The figure shows three views and two pictorial views of one solid part (mm, origin at its lowest corner). Answer the questions. A direction names the side the tool comes from. Round coordinates to 2 decimals unless told otherwise and drop trailing zeros. Write each loop counter-clockwise with the first axis right and the second up, starting at its lowest first coordinate (ties: lowest second). Pieces come first, ordered by that corner, then holes. Notation, with made-up numbers: (56, 46) - (72, 46) arc R16 ccw to (72, 50) - close; hole circle Ø2 at (73, -23). An arc over 180 degrees is marked (long way). Answer as CSV lines item,"result". Start each with the question number.
Item 1: A cutting plane is placed at C-C on x = 2.5. Determine the outline of the cut face in (y, z) (1 decimal).
Item 2: A cutting plane is placed at A-A on x = 5.75. Determine the outline of the cut face in (y, z) (1 decimal), and give its area (3 significant figures).
Item 3: Straight lines are drawn through the part: line 1 along Y through (x, z) = (6, 12.75); line 2 along Z through (x, y) = (6.75, 9.25); line 3 along Z through (x, y) = (2.5, 7.25) (1 decimal). For each, find the intervals that lie inside material, in ascending order. Write a range as [from, to].
Item 4: For a pull along Y with two mould halves and no side action, classify the marked faces 1, 2 and 3 as pulls with the +Y half, pulls with the -Y half, needs draft (parallel to the pull), parting line crosses it, or undercut.
Item 5: Flat-ended cylindrical pins translate along their axes: pin 1 (8 mm diameter, centred on y = 7, z = 16, fed in from +X); pin 2 (2 mm diameter, centred on x = 9.5, z = 15.5, fed in from -Y); pin 3 (4.5 mm diameter, centred on x = 6, y = 6.93, fed in from +Z). Find the tip coordinate at first contact, or state that the pin passes through.
Item 6: A cutting plane is placed at D-D on z = 5.5. Determine the outline of the cut face in (x, y).
Item 7: Which of the six approach directions +Z, -Z, +X, -X, +Y, -Y give full straight-line access (tool end or side, diameter ignored) to the marked faces 4 and 5?
Item 8: A cutting plane is placed at B-B on z = 14.3. Determine the outline of the cut face in (x, y).
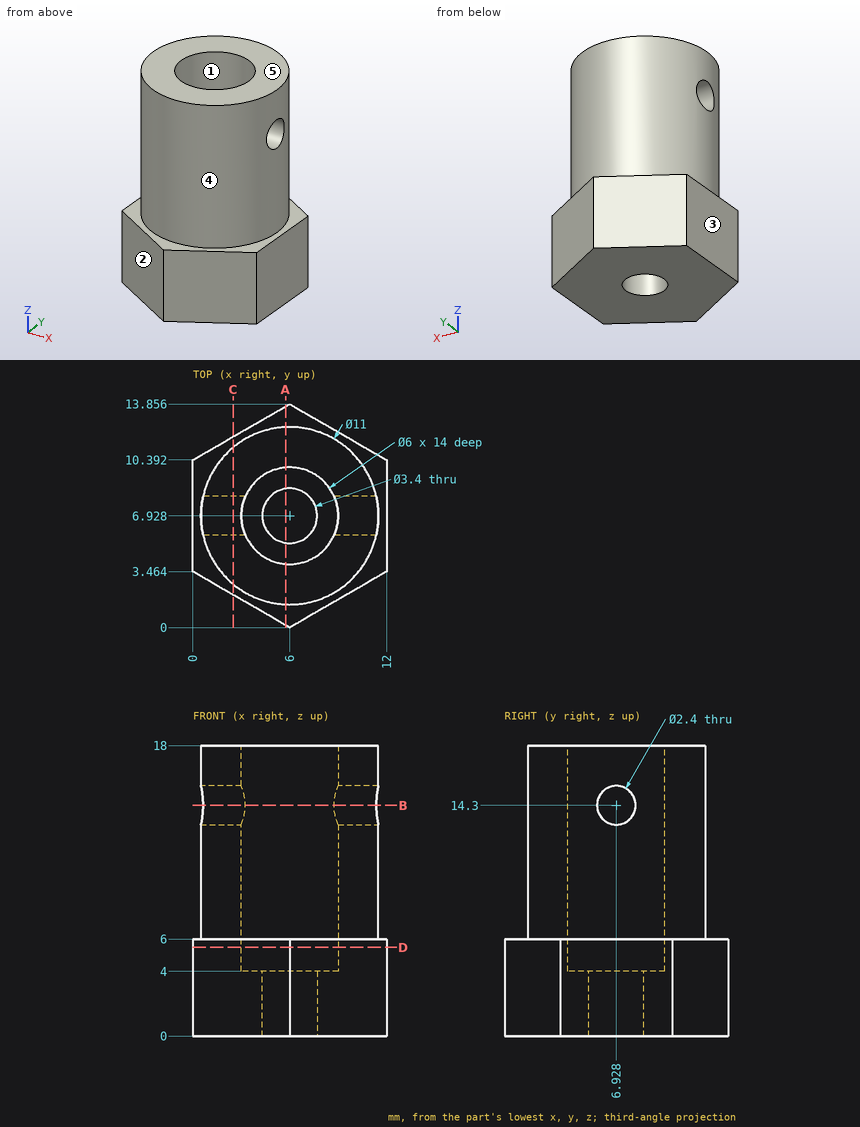
Geometry says:
1,outline,"(2, 0) - (11.8, 0) - (11.8, 6) - (11.2, 6) - (11.2, 18) - (2.7, 18) - (2.7, 6) - (2, 6) - close; hole circle Ø2.4 at (6.9, 14.3)"
2,outline,"(0.1, 0) - (5.2, 0) - (5.2, 4) - (3.9, 4) - (3.9, 18) - (1.4, 18) - (1.4, 6) - (0.1, 6) - close; (8.6, 0) - (13.7, 0) - (13.7, 6) - (12.4, 6) - (12.4, 18) - (9.9, 18) - (9.9, 4) - (8.6, 4) - close"
2,area,"116 mm^2"
3,line 1,"y = [1.43, 3.93], [9.93, 12.43]"
3,line 2,"z = [0, 4]"
3,line 3,"z = [0, 13.1], [15.5, 18]"
4,face 1,"undercut"
4,face 2,"pulls with the -Y half"
4,face 3,"needs draft"
5,pin 1,"stops at x = 11.5"
5,pin 2,"stops at y = 2.03"
5,pin 3,"stops at z = 4"
6,outline,"(0, 3.46) - (6, 0) - (12, 3.46) - (12, 10.39) - (6, 13.86) - (0, 10.39) - close; hole circle Ø6 at (6, 6.93)"
7,face 4,"+Z"
7,face 5,"+Z, +X, -X, +Y, -Y"
8,outline,"(0.63, 5.73) arc R5.5 ccw to (11.37, 5.73) - (8.75, 5.73) arc R3 cw to (3.25, 5.73) - close; (0.63, 8.13) - (3.25, 8.13) arc R3 cw to (8.75, 8.13) - (11.37, 8.13) arc R5.5 ccw to start"
